```python
from build123d import *

# Parameters (mm, degrees)
SKETCH1_R           = 11
SKETCH1_R_2         = 1
BOSS_EXTRUDE1_DEPTH = 3
SKETCH2_R           = 4
BOSS_EXTRUDE2_DEPTH = 15
SKETCH3_R           = 1.5
CUT_EXTRUDE1_DEPTH  = 5


with BuildPart() as part:
    # Sketch1 → Boss-Extrude1 (new body)
    with BuildSketch(Plane(origin=(0, 0, 0), x_dir=(1, 0, 0), z_dir=(0, 1, 0))):
        with Locations(Location((0, 0, 0), (0, 0, 270))):
            Circle(SKETCH1_R)
        with Locations(Location((0, 8, 0), (0, 0, 270))):
            Circle(SKETCH1_R_2, mode=Mode.SUBTRACT)
        with Locations(Location((8, 0, 0), (0, 0, 270))):
            Circle(SKETCH1_R_2, mode=Mode.SUBTRACT)
        with Locations(Location((0, -8, 0), (0, 0, 270))):
            Circle(SKETCH1_R_2, mode=Mode.SUBTRACT)
        with Locations(Location((-8, 0, 0), (0, 0, 270))):
            Circle(SKETCH1_R_2, mode=Mode.SUBTRACT)
    extrude(amount=BOSS_EXTRUDE1_DEPTH)

    # Sketch2 → Boss-Extrude2 (add)
    with BuildSketch(Plane(origin=(0, 3, 0), x_dir=(1, 0, 0), z_dir=(0, 1, 0))):
        with Locations(Location((0, 0, 0), (0, 0, 270))):
            Circle(SKETCH2_R)
    extrude(amount=BOSS_EXTRUDE2_DEPTH)

    # Sketch3 → Cut-Extrude1 (cut)
    with BuildSketch(Plane(origin=(0, 18, 0), x_dir=(1, 0, 0), z_dir=(0, 1, 0))):
        with Locations(Location((0, 0, 0), (0, 0, 270))):
            Circle(SKETCH3_R)
    extrude(amount=-CUT_EXTRUDE1_DEPTH, mode=Mode.SUBTRACT)


solid = part.part
```
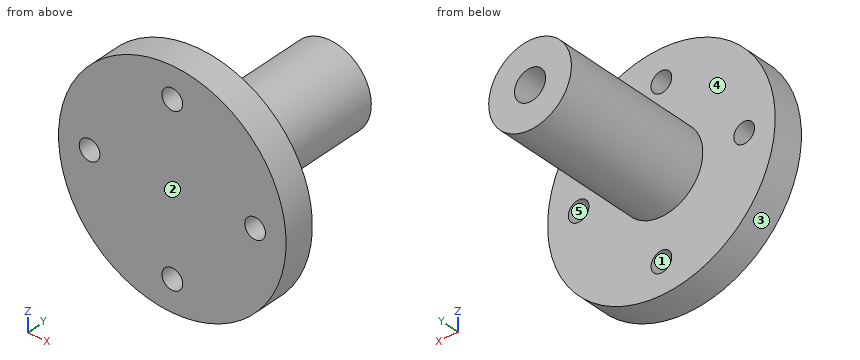
For this review, take the finished solid that the model builds, in its own axes (mm). Face numbers are marked on the shaded views. A direction names the side the tool comes from. Give positions to 0.01 mm unless a question says otherwise; leave off trailing zeros. Write each loop counter-clockwise with the first axis right and the second up, starting at its lowest first coordinate (ties: lowest second). Pieces come first, ordered by that corner, then holes.
Item 1: Machinability: for the marked faces 4 and 5, which of the approach directions +Z, -Z, +X, -X, +Y, -Y give a long, thin tool a straight path to every point of the face, cutting with its end or side? Answer none if there is none.
Item 2: Take a section at D-D (x = -8). Give the boundary of the cut face in (y, z), and give its area (3 significant figures).
Item 3: Wall thickness on probe 1 along X at (y, z) = (16.8, 0); probe 2 along Y at (x, z) = (9.25, -1); probe 3 along X at (y, z) = (1.4, 8): over which ranges is each line inside the solid? List them lowest first.
Item 4: Take a section at C-C (z = 8). Give the boundary of the cut face in (x, y), and give its area (3 significant figures).
Item 5: Take a section at A-A (x = 0). Give the boundary of the cut face in (y, z).
Item 6: Insertion check: P1, Ø1.2, axis at x = 0, z = 8, coming from the -Y side; P2, Ø2.5, axis at x = -8, z = 0, coming from the -Y side; P3, Ø5, axis at x = -7, z = 8, coming from the +Y side; P4, Ø5, axis at x = -3.5, y = 12.5, coming from the +Z side. Each pin has a flat end and moves straight along its axis. Give the tip position at first contact, or say it passes through.
Item 7: Take a section at B-B (z = 0). Give the boundary of the cut face in (x, y).
Item 8: The part is to be moulded in two halves that separate along X. For the marked faces 1, 2 and 3, say which applies: +X half, -X half, draft (parallel to the pull), parting line (faces both ways), or undercut.
Established:
1. face 4: +Y
1. face 5: +Y, -Y
2. outline: (0, -7.55) - (3, -7.55) - (3, -1) - (0, -1) - close; (0, 1) - (3, 1) - (3, 7.55) - (0, 7.55) - close
2. area: 39.3 mm2
3. probe 1: x = -4 to -1.5, 1.5 to 4
3. probe 2: y = 0 to 3
3. probe 3: x = -7.55 to -1, 1 to 7.55
4. outline: (-7.55, 0) - (-1, 0) - (-1, 3) - (-7.55, 3) - close; (1, 0) - (7.55, 0) - (7.55, 3) - (1, 3) - close
4. area: 39.3 mm2
5. outline: (0, -11) - (3, -11) - (3, -9) - (0, -9) - close; (0, -7) - (3, -7) - (3, -4) - (18, -4) - (18, -1.5) - (13, -1.5) - (13, 1.5) - (18, 1.5) - (18, 4) - (3, 4) - (3, 7) - (0, 7) - close; (0, 9) - (3, 9) - (3, 11) - (0, 11) - close
6. P1: passes through
6. P2: stops at y = 0
6. P3: stops at y = 3
6. P4: stops at z = 3.87
7. outline: (-11, 0) - (-9, 0) - (-9, 3) - (-11, 3) - close; (-7, 0) - (7, 0) - (7, 3) - (4, 3) - (4, 18) - (1.5, 18) - (1.5, 13) - (-1.5, 13) - (-1.5, 18) - (-4, 18) - (-4, 3) - (-7, 3) - close; (9, 0) - (11, 0) - (11, 3) - (9, 3) - close
8. face 1: undercut
8. face 2: draft
8. face 3: parting line
